Here's the drawing with two shaded views (mm, measured from the low corner). I have some questions. A direction names the side the tool comes from. Coordinates: 2 decimals unless noted, no trailing zeros. Write each loop counter-clockwise with the first axis right and the second up, starting at its lowest first coordinate (ties: lowest second). Pieces come first, ordered by that corner, then holes.
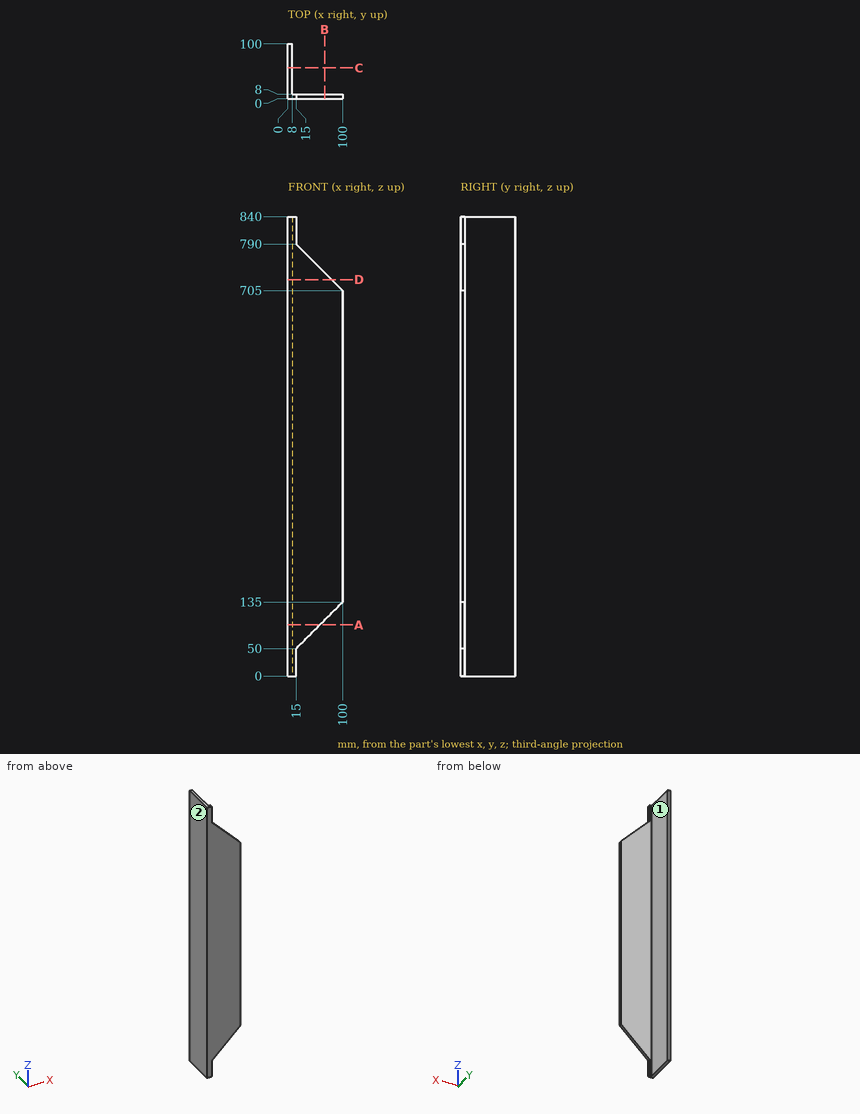
Item 1: I want a section at C-C, the plane y = 56.5. List the corners of the cut face in (x, z) for me.
Item 2: I want a section at A-A, the plane z = 93.5. List the corners of the cut face in (x, y) for me, then the cut area to 3 significant figures.
Item 3: I want a section at D-D, the plane z = 725. List the corners of the cut face in (x, y) for me, then the cut area to 3 significant figures.
Item 4: If I drill on line 1 along Y through (x, z) = (36.5, 489); line 2 along Z through (x, y) = (83.5, 7), over which ranges is the centre line in solid material (lowest first)?
Item 5: Will these pins go through, and if not, where does the flat tip stop? pin 1 Ø12 at (x, z) = (69, 685.5) entering from +Y; pin 2 Ø4 at (y, z) = (5, 822.5) entering from +X; pin 3 Ø6 at (y, z) = (22.5, 103.5) entering from +X.
Item 6: I want a section at B-B, the plane x = 67.5. List the corners of the cut face in (y, z) for me.
Item 7: Which directions (+Z, -Z, +X, -X, +Y, -Y) give clear straight access to the entire face, cutting with the end or side of a thin tool? Please do the marked faces 1 and 2.
Taken from the geometry:
1. outline: (0, 0) - (8, 0) - (8, 840) - (0, 840) - close
2. outline: (0, 0) - (58.5, 0) - (58.5, 8) - (8, 8) - (8, 100) - (0, 100) - close
2. area: 1,200 mm2
3. outline: (0, 0) - (80, 0) - (80, 8) - (8, 8) - (8, 100) - (0, 100) - close
3. area: 1,380 mm2
4. line 1: y = 0 to 8
4. line 2: z = 118.5 to 721.5
5. pin 1: stops at y = 8
5. pin 2: stops at x = 15
5. pin 3: stops at x = 8
6. outline: (0, 102.5) - (8, 102.5) - (8, 737.5) - (0, 737.5) - close
7. face 1: +Z, -Z, +X, +Y
7. face 2: +Z, -Z, -X, +Y, -Y
